from build123d import *

# Parameters (mm, degrees)
SKETCH_1_W          = 2252
SKETCH_1_H          = 100
SKETCH_1_R          = 13
EXTRUDE_1_DEPTH     = 8
SKETCH_2_W          = 2252
SKETCH_2_H          = 8
EXTRUDE_2_DEPTH     = 92
CHAMFER_3_SIZE      = 25
CHAMFER_4_SIZE      = 25
CUT_EXTRUDE_3_DEPTH = 1135.846245092
CHAMFER_5_SIZE      = 25
CHAMFER_6_SIZE      = 25


with BuildPart() as part:
    # 草图1 → 凸台-拉伸1 (new body)
    with BuildSketch(Plane.XY):
        with Locations((0, 50)):
            Rectangle(SKETCH_1_W, SKETCH_1_H)
        with Locations((1086, 50)):
            Circle(SKETCH_1_R, mode=Mode.SUBTRACT)
        with Locations((971, 50)):
            Circle(SKETCH_1_R, mode=Mode.SUBTRACT)
        with Locations((0, 50)):
            Circle(SKETCH_1_R, mode=Mode.SUBTRACT)
        with Locations((80, 50)):
            Circle(SKETCH_1_R, mode=Mode.SUBTRACT)
        with Locations((160, 50)):
            Circle(SKETCH_1_R, mode=Mode.SUBTRACT)
        with Locations(Location((-80, 50, 0), (0, 0, 180))):
            Circle(SKETCH_1_R, mode=Mode.SUBTRACT)
        with Locations(Location((-160, 50, 0), (0, 0, 180))):
            Circle(SKETCH_1_R, mode=Mode.SUBTRACT)
        with Locations(Location((-971, 50, 0), (0, 0, 180))):
            Circle(SKETCH_1_R, mode=Mode.SUBTRACT)
        with Locations(Location((-1086, 50, 0), (0, 0, 180))):
            Circle(SKETCH_1_R, mode=Mode.SUBTRACT)
    extrude(amount=EXTRUDE_1_DEPTH)

    # 草图2 → 凸台-拉伸2 (add)
    with BuildSketch(Plane.XY.offset(8)):
        with Locations((0, 96)):
            Rectangle(SKETCH_2_W, SKETCH_2_H)
    extrude(amount=EXTRUDE_2_DEPTH)

    # 倒角3
    chamfer_3_edges = [part.edges().sort_by_distance(p)[0] for p in [
        (1126, 0, 4),
    ]]
    chamfer(chamfer_3_edges, length=CHAMFER_3_SIZE)

    # 倒角4
    chamfer_4_edges = [part.edges().sort_by_distance(p)[0] for p in [
        (1126, 100, 50),
    ]]
    chamfer(chamfer_4_edges, length=CHAMFER_4_SIZE)

    # 草图3 → 切除-拉伸3 (cut, through all)
    with BuildSketch(Plane(origin=(0, 100, 0), x_dir=(1, 0, 0), z_dir=(0, 1, 0))):
        Polygon((886, -100), (1126, 0), (1126, -100), align=None)
    cut_extrude_3 = extrude(amount=-CUT_EXTRUDE_3_DEPTH, mode=Mode.SUBTRACT)

    # 倒角5
    chamfer_5_edges = [part.edges().sort_by_distance(p)[0] for p in [
        (-1126, 0, 4),
    ]]
    chamfer(chamfer_5_edges, length=CHAMFER_5_SIZE)

    # 倒角6
    chamfer_6_edges = [part.edges().sort_by_distance(p)[0] for p in [
        (-1126, 100, 50),
    ]]
    chamfer(chamfer_6_edges, length=CHAMFER_6_SIZE)

    # 镜向8: 切除-拉伸3 across plane
    add(cut_extrude_3.mirror(Plane(origin=(0, 0, 0), x_dir=(0, 0, 1), z_dir=(1, 0, 0))), mode=Mode.SUBTRACT)


solid = part.part
Input: part model. Units: mm. Frame: model coordinates. A direction names the side the tool comes from. Coordinates: 2 decimals unless noted, no trailing zeros. Loops run counter-clockwise (first coordinate to the right, second up) from the corner with the lowest first, then second, coordinate; pieces in that order, holes last. Notation, with made-up numbers: (74, -26) -> (106, -26) arc R24 ccw to (106, 9) -> close; hole circle Ø11 at (-39, -22). An arc over 180 degrees is marked (long way). One line per item, written item: value.
(1) Set-up query: faces 1 (the face through (-15, 47, 8)), 2 (the face through (-15, 100, 49)). Return all of +Z, -Z, +X, -X, +Y, -Y with unobstructed straight access to the full face (end or side cutting, diameter ignored); none if empty.
Answer below:
face 1: +Z, +X, -X, -Y
face 2: +Z, -Z, +X, -X, +Y
(2) Cut plane A-A (x = 554). Output: boundary loops of the cut face in (y, z), then the cut area to 3 significant figures.
Answer below:
outline: (0, 0) -> (100, 0) -> (100, 100) -> (92, 100) -> (92, 8) -> (0, 8) -> close
area: 1,540 mm2
(3) Pin query (flat end, axial travel): pin 1 Ø15.5 at (x, y) = (971, 50) entering from -Z; pin 2 Ø2 at (x, z) = (9.5, 51) entering from -Y. Return the tip coordinate at first contact, or that it passes through.
Answer below:
pin 1: passes through
pin 2: stops at y = 92
(4) Cut plane B-B (z = 28). Output: boundary loops of the cut face in (x, y), then the cut area to 3 significant figures.
Answer below:
outline: (-1058.8, 92) -> (1058.8, 92) -> (1058.8, 100) -> (-1058.8, 100) -> close
area: 16,900 mm2
(5) Ray query, line 1 along Y through (x, z) = (-160, 5); line 2 along Y through (x, z) = (327, 19); line 3 along Z through (x, y) = (-950.5, 43.5). Return the intervals inside material, ascending.
Answer below:
line 1: y = 0 to 37, 63 to 100
line 2: y = 92 to 100
line 3: z = 0 to 8
